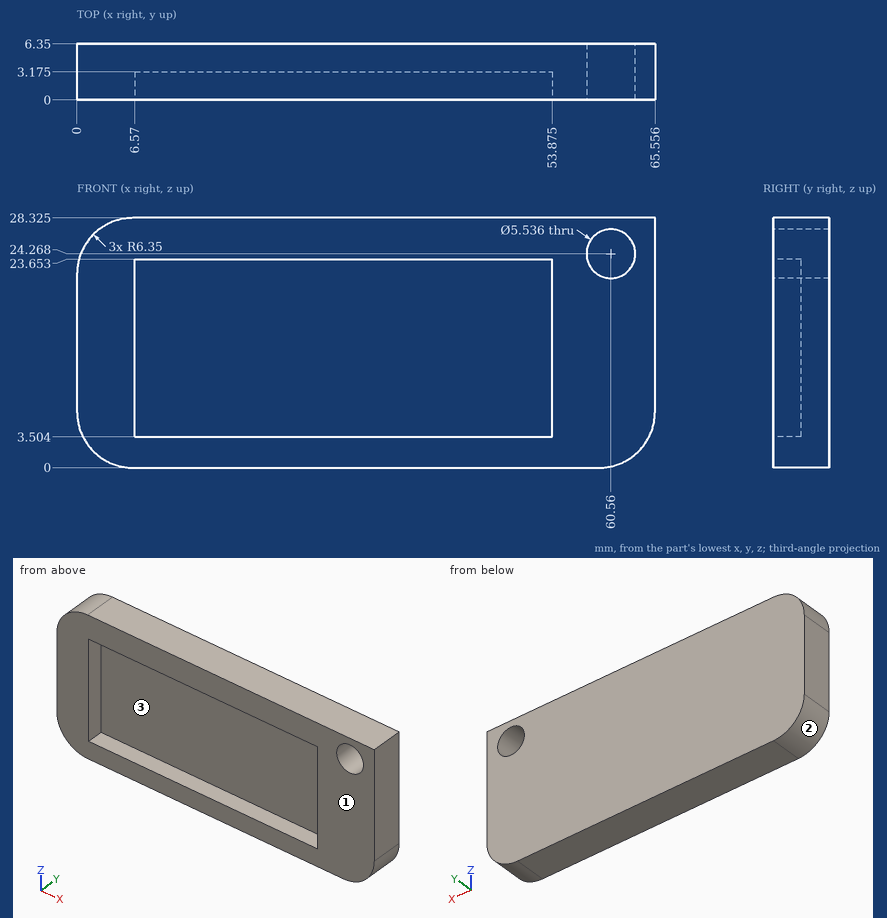
Job drawing, mm, ordinate dimensions from the low corner. One solid piece. Coordinates: 2 decimals unless noted, no trailing zeros. Answer in a Markdown table with one row per item. Add a question column.
Q1. Wall check: line 1 along Z through (x, y) = (39, 3) (1 decimal); line 2 along X through (y, z) = (3.75, 6.25) (1 decimal); line 3 along X through (y, z) = (1.5, 18) (1 decimal). Give the ranges that are in metal, low to high. Write a range as [from, to].
Q2. Mould opens along X. For the marked faces 1, 2 and 3 say: +X half, -X half, draft (parallel to the pull), parting line (faces both ways), or undercut.
Q3. Drop flat-ended pins along their axis: pin 1 (3 mm diameter, centred on x = 50.5, z = 16.5, fed in from -Y) (1 decimal); pin 2 (3 mm diameter, centred on y = 5.5, z = 4.5, fed in from -X); pin 3 (5 mm diameter, centred on x = 60.56, z = 24.27, fed in from -Y). Give the stop position or say it passes through.
Answers follow:
| question | item | result |
|---|---|---|
| 1 | line 1 | [0, 3.5], [23.7, 28.3] |
| 1 | line 2 | [0, 65.6] |
| 1 | line 3 | [0, 6.6], [53.9, 65.6] |
| 2 | face 1 | draft |
| 2 | face 2 | -X half |
| 2 | face 3 | undercut |
| 3 | pin 1 | y = 3.2 |
| 3 | pin 2 | x = 0.01 |
| 3 | pin 3 | through |
